Check sheet for the modelled part. Datum: model origin and axes. Units: mm. A direction names the side the tool comes from. Coordinates: 2 decimals unless noted, no trailing zeros. Write each question's results on one line, items separated by ' | '. Start each with the question number.
1. Thickness scan on line 1 (Y direction, x = 30, z = 12.25); line 2 (Y direction, x = 91, z = 14.25); line 3 (X direction, y = 55, z = 12.25). Record the ranges inside material, lowest first. Write a range as [from, to].
2. Gauge pin test, flat ends, axial feed: P1, Ø4.5, axis at x = -50, z = 9, coming from the -Y side; P2, Ø5, axis at x = -70, y = 0, coming from the -Z side. Record the tip position at first contact, or that the pin passes through.
3. Draft check along Y on faces 4 (the face through (-100, -3, 9)), 5 (the face through (30.521, -176.034, 8.874)), 6 (the face through (91.867, 51.095, 10.395)), 7 (the face through (0.09, -206.014, 8.311)). Enter one of: released by +Y, released by -Y, zero draft, split by the parting line, or undercut.
4. Tool access check on faces 1 (the face through (-1, 3, 0)), 2 (the face through (91.521, 158.966, 10.395)), 3 (the face through (-0.867, -218.846, 12.905)). Record the directions out of +Z, -Z, +X, -X, +Y, -Y that give a thin tool (end or side, any length) a straight path to the whole face; none if there is none.
```python
from build123d import *

# Parameters (mm, degrees)
SKETCH1_W                  = 200
SKETCH1_H                  = 460
BOSS_EXTRUDE1_DEPTH        = 18
OTWORY_USTALAJ_CE_8_0MM1_D = 8
OTW_R_7_0_7_1_D            = 7
OTW_R_5_0_5_1_D            = 5
OTW_R_5_0_5_1_DEPTH        = 45
OTW_R_5_0_5_1_TIP          = 1.502151548
OTW_R_8_0_8_1_D            = 8
OTW_R_8_0_8_1_DEPTH        = 15
OTW_R_8_0_8_1_TIP          = 2.403442476
OTW_R_8_0_8_2_D            = 8
OTW_R_8_0_8_2_DEPTH        = 22
OTW_R_8_0_8_2_TIP          = 2.403442476


with BuildPart() as part:
    # Sketch1 → Boss-Extrude1 (new body)
    with BuildSketch(Plane.XY):
        Rectangle(SKETCH1_W, SKETCH1_H)
    extrude(amount=BOSS_EXTRUDE1_DEPTH)

    # Otwory ustalające Ø8.0mm1 (through all)
    with Locations(Plane.XY.offset(18)):
        with Locations((30, -180), (-70, -180), (-70, 0), (30, 0), (30, 180), (-70, 180)):
            Hole(OTWORY_USTALAJ_CE_8_0MM1_D / 2)

    # Otwór Ø7.0 (7)1 (through all)
    with Locations(Plane.XY.offset(18)):
        with Locations((91, 30), (91, 180)):
            Hole(OTW_R_7_0_7_1_D / 2)

    # Otwór Ø5.0 (5)1
    with Locations(Plane(origin=(0, -230, 0), x_dir=(-1, 0, 0), z_dir=(0, -1, 0))):
        with Locations((-50, -9), (50, -9)):
            Hole(OTW_R_5_0_5_1_D / 2, depth=OTW_R_5_0_5_1_DEPTH)
            with Locations((0, 0, -(OTW_R_5_0_5_1_DEPTH + OTW_R_5_0_5_1_TIP / 2))):  # 118° drill point
                Cone(0, OTW_R_5_0_5_1_D / 2, OTW_R_5_0_5_1_TIP, mode=Mode.SUBTRACT)

    # Otwór Ø8.0 (8)1
    with Locations(Plane.XY.offset(18)):
        with Locations((91, 55), (91, 155)):
            Hole(OTW_R_8_0_8_1_D / 2, depth=OTW_R_8_0_8_1_DEPTH)
            with Locations((0, 0, -(OTW_R_8_0_8_1_DEPTH + OTW_R_8_0_8_1_TIP / 2))):  # 118° drill point
                Cone(0, OTW_R_8_0_8_1_D / 2, OTW_R_8_0_8_1_TIP, mode=Mode.SUBTRACT)

    # Otwór Ø8.0 (8)2
    with Locations(Plane(origin=(0, -230, 0), x_dir=(-1, 0, 0), z_dir=(0, -1, 0))):
        with Locations((0, -9)):
            Hole(OTW_R_8_0_8_2_D / 2, depth=OTW_R_8_0_8_2_DEPTH)
            with Locations((0, 0, -(OTW_R_8_0_8_2_DEPTH + OTW_R_8_0_8_2_TIP / 2))):  # 118° drill point
                Cone(0, OTW_R_8_0_8_2_D / 2, OTW_R_8_0_8_2_TIP, mode=Mode.SUBTRACT)


solid = part.part
```
Established:
1) line 1: [-230, -184], [-176, -4], [4, 176], [184, 230] | line 2: [-230, 26.5], [33.5, 51], [59, 151], [159, 176.5], [183.5, 230] | line 3: [-100, 87], [95, 100]
2) P1: y = -184.85 | P2: through
3) face 4: zero draft | face 5: undercut | face 6: undercut | face 7: released by -Y
4) face 1: -Z, +X, -X, +Y, -Y | face 2: +Z | face 3: -Y
